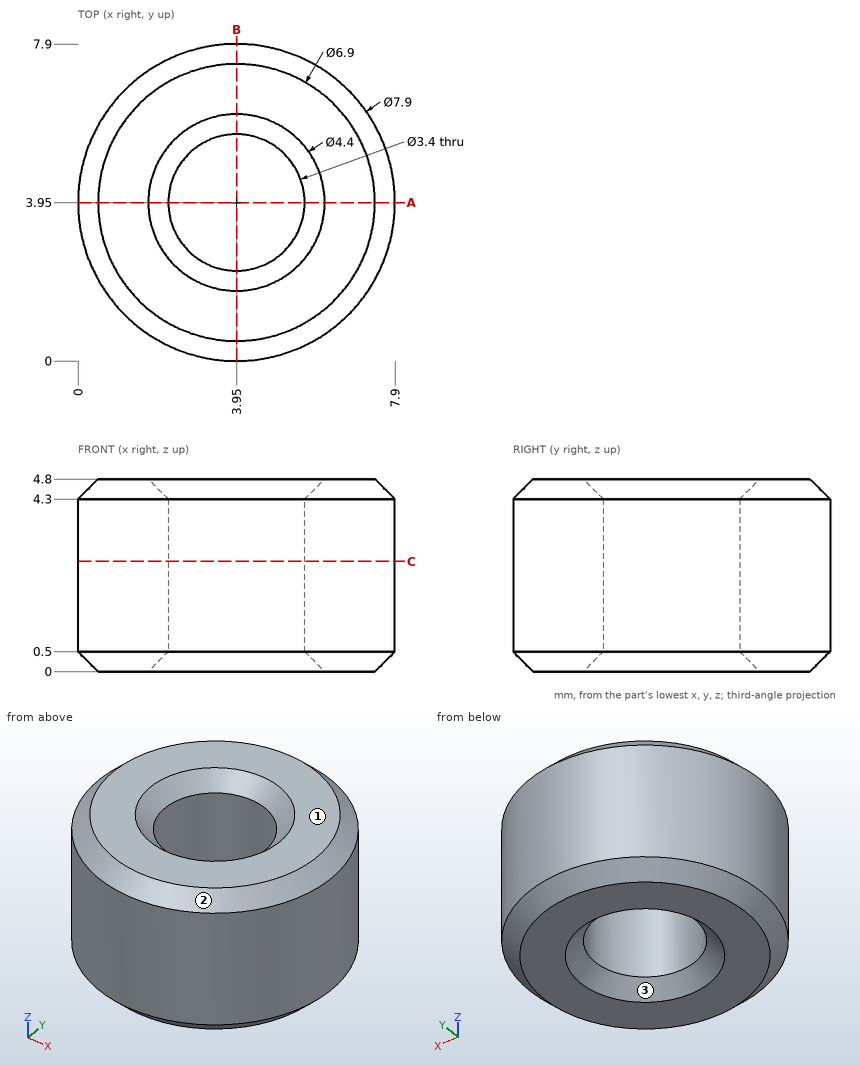
Job drawing, mm, ordinate dimensions from the low corner. One solid piece. Give positions to 0.01 mm unless a question says otherwise; leave off trailing zeros. Order: outer loops, then holes, each group sorted by start corner. A loop starts at its lowest first (then second) coordinate and runs counter-clockwise, first axis right, second up. Notation, with made-up numbers: M 50,-7.5 L 105,-7.5 A23 cw 105,26.5 Z; hole C -15.5,65 d1. An arc over 180 degrees is marked long. Put each result on its own line as item: value. Start each with the question number.
(1) Pin check, flat tips, straight feed: pin 1 Ø1 at (y, z) = (6, 3) entering from +X; pin 2 Ø1 at (x, y) = (2.5, 4.5) entering from +Z; pin 3 Ø2 at (x, z) = (2.5, 1) entering from +Y. Stop position of each tip, or through.
(2) Drill centre lines: L1, parallel to Y at x = 3.95, z = 2.65; L2, parallel to X at y = 2.75, z = 3.4; L3, parallel to X at y = 5.5, z = 1.25. Where is each one in solid material? Low to high. Write a range as [from, to].
(3) Band-saw the part on C-C on z = 2.75. Give the cut face in (x, y), then the cut area to 3 significant figures.
(4) Pull direction X, two halves, no side cores. Call the marked faces 1, 2 and 3: released by +X, released by -X, zero draft, split by the parting line, or undercut.
(5) Band-saw the part on A-A on y = 3.95. Give the cut face in (x, z), then the cut area to 3 significant figures.
Results below:
1. pin 1: stops at x = 7.58
1. pin 2: stops at z = 4.65
1. pin 3: stops at y = 7.87
2. L1: y = [0, 2.25], [5.65, 7.9]
2. L2: x = [0.19, 2.75], [5.15, 7.71]
2. L3: x = [0.32, 3.25], [4.65, 7.58]
3. outline: C 3.95,3.95 d7.9; hole C 3.95,3.95 d3.4
3. area: 39.9 mm2
4. face 1: zero draft
4. face 2: split by the parting line
4. face 3: undercut
5. outline: M 0,0.5 L 0.5,0 L 1.75,0 L 2.25,0.5 L 2.25,4.3 L 1.75,4.8 L 0.5,4.8 L 0,4.3 Z; M 5.65,0.5 L 6.15,0 L 7.4,0 L 7.9,0.5 L 7.9,4.3 L 7.4,4.8 L 6.15,4.8 L 5.65,4.3 Z
5. area: 20.6 mm2
